Model file for the job. Use its own axes, mm. A direction names the side the tool comes from. Give positions to 0.01 mm unless a question says otherwise; leave off trailing zeros. Write each loop counter-clockwise with the first axis right and the second up, starting at its lowest first coordinate (ties: lowest second). Pieces come first, ordered by that corner, then holes. Notation, with made-up numbers: (-28, 66.5) - (-17, 66.5) arc R26 ccw to (-17, 89.5) - close; hole circle Ø9 at (45.25, -20.5). An arc over 180 degrees is marked (long way). Use a Markdown table: item, result. Add a question column.
Autodesk Inventor part; units mm, degrees
ref_plane "YZ Plane" through (0, 0, 0) normal (1, 0, 0) x (0, 1, 0)
ref_plane "XZ Plane" through (0, 0, 0) normal (0, 1, 0) x (-1, 0, 0)
ref_plane "XY Plane" through (0, 0, 0) normal (0, 0, 1) x (1, 0, 0)
sketch "Skizze1" plane through (0, 0, 0) normal (0, 0, 1) x (1, 0, 0)
  circle A0 centre (0, 0) radius 17.5
  circle A1 centre (0, 0) radius 12.5 construction
  line L0 (-4, 11.8427) -> (4, 11.8427) construction
  line L1 (4, 11.8427) -> (4, -11.8427)
  line L2 (4, -11.8427) -> (-4, -11.8427) construction
  line L3 (-4, -11.8427) -> (-4, 11.8427)
  arc A2 (-4, 11.8427) -> (-4, -11.8427) centre (0, 0) ccw
  arc A3 (4, -11.8427) -> (4, 11.8427) centre (0, 0) ccw
  dimension "d0" = 35
  dimension "d1" = 25
  dimension "d2" = 8
  dimension "d3" = 4
  dimension "d4" = 25
  dimension "d5" = 0
extrude "Extrusion1" add sketch "Skizze1" along normal blind 10
sketch "Skizze2" plane through (4, -11.8427, 0) normal (1, 0, 0) x (0, 0, -1)
  circle A0 centre (-5, 15.6854) radius 2.525
  circle A1 centre (-5, 8) radius 2.525
  line L0 (0, 0) -> (-10, 0)
  line L1 (0, 23.6854) -> (-10, 23.6854)
  line L2 (-10, 0) -> (-10, 23.6854)
  point P0 (0, 11.8427)
  dimension "d8" = 5.05
  dimension "d9" = 5.05
  dimension "d10" = 8
  dimension "d11" = 8
  dimension "d12" = 5
  dimension "d13" = 5
extrude "Extrusion2" cut sketch "Skizze2" along normal mid plane 500
sketch "Skizze3" plane through (0, 0, 10) normal (0, 0, 1) x (1, 0, 0)
  circle A0 centre (0, 0) radius 12.55
  line L0 (4, 11.8955) -> (4, -11.8955)
  line L1 (-4, -11.8955) -> (-4, 11.8955)
  dimension "d16" = 25.1
  dimension "d17" = 4
  dimension "d18" = 8
extrude "Extrusion3" cut sketch "Skizze3" against normal through all contours A0 L0 | L1 A0
properties part number "FahnenhalterTeiloben"
(1) Flat gauge pins, fed straight in: pin 1 (2 mm diameter, centred on y = 6.5, z = 3.5, fed in from +X); pin 2 (1 mm diameter, centred on x = -8, z = 2, fed in from -Y); pin 3 (3 mm diameter, centred on y = 3, z = 7, fed in from +X). Where does each tip first touch, or does it go through?
(2) Probe probe 1 along X at (y, z) = (-6.5, 4.5); probe 2 along Z at (x, y) = (15.5, -4); probe 3 along X at (y, z) = (10, 4.25). List the from-to ranges inside material, lowest first. Write a range as [from, to].
(3) Which spindle directions (+Z, -Z, +X, -X, +Y, -Y) get a long thin tool onto all of the face, cutting with end or side? Do faces 4 (the cylindrical face through (0.056, -4.81, 2.668)), 5 (the flat face through (-4, 0, 5)). Say none if no direction does.
(4) Band-saw the part on B-B (z = 6). Write the cut outline in (x, y), then the cut area to 3 significant figures.
(5) Band-saw the part on C-C (x = 8). Write the cut outline in (y, z).
(6) Band-saw the part on D-D (y = -4.5). Write the cut outline in (x, z).
(7) Two-plate mould, pull along Y, no slides. Class faces 1 (the flat face through (0, 0, 10)), 2 (the cylindrical face through (-14.09, 5.97, 3.64)), 3 (the cylindrical face through (-13.887, 10.648, 4.93)): +Y half, -Y half, draft (parallel to the pull), parting line (faces both ways), or undercut.
(8) Band-saw the part on A-A (y = 0). Write the cut outline in (x, z), then the cut area to 3 significant figures.
Model answer:
| question | item | result |
|---|---|---|
| 1 | pin 1 | stops at x = 16.59 |
| 1 | pin 2 | stops at y = -15.81 |
| 1 | pin 3 | stops at x = 17.44 |
| 2 | probe 1 | x = [-16.25, -10.74], [-4, 4], [10.74, 16.25] |
| 2 | probe 2 | z = [0, 2.48], [7.52, 10] |
| 2 | probe 3 | x = [-14.36, -7.58], [-4, 4], [7.58, 14.36] |
| 3 | face 4 | +X, -X |
| 3 | face 5 | +Z, -Z |
| 4 | outline | (-17.43, -1.52) - (-12.46, -1.52) arc R12.55 cw to (-12.46, 1.52) - (-17.43, 1.52) arc R17.5 ccw to start; (-16.38, -6.16) arc R17.5 ccw to (16.38, -6.16) - (10.93, -6.16) arc R12.55 cw to (4, -11.9) - (4, -6.16) - (-4, -6.16) - (-4, -11.9) arc R12.55 cw to (-10.93, -6.16) - close; (-16.38, 6.16) - (-10.93, 6.16) arc R12.55 cw to (-4, 11.9) - (-4, 6.16) - (4, 6.16) - (4, 11.9) arc R12.55 cw to (10.93, 6.16) - (16.38, 6.16) arc R17.5 ccw to start; (-4, -1.52) - (4, -1.52) - (4, 1.52) - (-4, 1.52) - close; (12.46, -1.52) - (17.43, -1.52) arc R17.5 ccw to (17.43, 1.52) - (12.46, 1.52) arc R12.55 cw to start |
| 4 | area | 495 mm^2 |
| 5 | outline | (-15.56, 0) - (-9.67, 0) - (-9.67, 10) - (-15.56, 10) - close; (9.67, 0) - (15.56, 0) - (15.56, 10) - (9.67, 10) - close |
| 6 | outline | (-16.91, 0) - (-11.72, 0) - (-11.72, 2.56) - (-16.91, 2.56) - close; (-16.91, 7.44) - (-11.72, 7.44) - (-11.72, 10) - (-16.91, 10) - close; (-4, 0) - (4, 0) - (4, 2.56) - (-4, 2.56) - close; (-4, 7.44) - (4, 7.44) - (4, 10) - (-4, 10) - close; (11.72, 0) - (16.91, 0) - (16.91, 2.56) - (11.72, 2.56) - close; (11.72, 7.44) - (16.91, 7.44) - (16.91, 10) - (11.72, 10) - close |
| 7 | face 1 | draft |
| 7 | face 2 | undercut |
| 7 | face 3 | parting line |
| 8 | outline | (-17.5, 0) - (-12.55, 0) - (-12.55, 10) - (-17.5, 10) - close; (-4, 0) - (4, 0) - (4, 10) - (-4, 10) - close; (12.55, 0) - (17.5, 0) - (17.5, 10) - (12.55, 10) - close |
| 8 | area | 179 mm^2 |
